from build123d import *

# Parameters (mm, degrees)
SKETCH1_R           = 2
BOSS_EXTRUDE1_DEPTH = 3
SKETCH2_R           = 5.5
SKETCH2_R_2         = 4
BOSS_EXTRUDE2_DEPTH = 0.5
SKETCH4_R           = 4
CUT_EXTRUDE2_DEPTH  = 7


with BuildPart() as part:
    # Sketch1 → Boss-Extrude1 (new body, symmetric)
    with BuildSketch(Plane.XY):
        with BuildLine():
            Line((-5.5, 0), (-14.456832295, -4))
            ThreePointArc((-14.456832295, -4), (0, -15), (14.456832295, -4))
            Line((14.456832295, -4), (5.5, 0))
            ThreePointArc((5.5, 0), (5.475559526, 0.517926522), (5.402455316, 1.03125))
            Line((5.402455316, 1.03125), (3.929058411, 8.75))
            ThreePointArc((3.929058411, 8.75), (0, 12), (-3.929058411, 8.75))
            Line((-3.929058411, 8.75), (-5.402455316, 1.03125))
            ThreePointArc((-5.402455316, 1.03125), (-5.475559526, 0.517926522), (-5.5, 0))
        make_face()
        with Locations((0, 8)):
            Circle(SKETCH1_R, mode=Mode.SUBTRACT)
    extrude(amount=BOSS_EXTRUDE1_DEPTH, both=True)

    # Sketch2 → Boss-Extrude2 (add)
    with BuildSketch(Plane.XY.offset(3)):
        Circle(SKETCH2_R)
        Circle(SKETCH2_R_2, mode=Mode.SUBTRACT)
    extrude(amount=BOSS_EXTRUDE2_DEPTH)

    # Sketch4 → Cut-Extrude2 (cut, through all)
    with BuildSketch(Plane.XY.offset(3)):
        Circle(SKETCH4_R)
    extrude(amount=-CUT_EXTRUDE2_DEPTH, mode=Mode.SUBTRACT)

    # Sketch8 → M4 Tapped Hole1 (revolve, cut)
    with BuildSketch(Plane(origin=(0, 0, 0), x_dir=(0, 0, 1), z_dir=(1, 0, 0))):
        Polygon((0, 0), (0, 22.491420021), (1.65, 21.5), (1.65, 0), align=None)
    revolve(axis=Axis((0, 6.35, 0), (0, -1, 0)), mode=Mode.SUBTRACT)


solid = part.part
Check sheet for the modelled part. Datum: model origin and axes. Units: mm. Give positions to 0.01 mm unless a question says otherwise; leave off trailing zeros. Loops run counter-clockwise (first coordinate to the right, second up) from the corner with the lowest first, then second, coordinate; pieces in that order, holes last. Notation, with made-up numbers: M 15,35 L 26,35 A12 ccw 26,51 Z; hole C 17.25,62 d5. An arc over 180 degrees is marked long. Return JSON: item names as keys, results as strings. Group by question number.
1. Cross-section at C-C on y = -0.75. Record the boundary of the cut face in (x, z), plus the area to 3 significant figures.
2. Cross-section at A-A on x = 0. Record the boundary of the cut face in (y, z), plus the area to 3 significant figures.
3. Mould release check, pull along Z, two halves, no side actions. Record for faces 1 (the flat face through (-0.2, -4.3, -3)), 2 (the cylindrical face through (-1.115, -9.244, -1.216)), 3 (the cylindrical face through (0, 10, 0)), 4 (the flat face through (1, 6, 3)): released by +Z, released by -Z, zero draft, split by the parting line, or undercut.
4. Go/stop test with flat-tipped pins: pin 1 (1.5 mm diameter, centred on x = -3.5, z = 2.5, fed in from +Y); pin 2 (1.5 mm diameter, centred on x = -4.5, z = 1.5, fed in from -Y); pin 3 (4.5 mm diameter, centred on x = -7, y = -10.5, fed in from +Z); pin 4 (6.5 mm diameter, centred on x = 0, y = 0, fed in from +Z). Record where each tip stops, or that it passes through.
5. Cross-section at D-D on z = 0. Record the boundary of the cut face in (x, y).
6. Cross-section at B-B on z = 2.25. Record the boundary of the cut face in (x, y).
7. Thickness scan on L1, parallel to Y at x = 0.5, z = -2.5; L2, parallel to Z at x = 0, y = -9.75; L3, parallel to Y at x = 0, z = -0.35. Record the ranges inside material, lowest first.
Return value:
{
 "1": {"outline": "M -7.18,-3 L -3.93,-3 L -3.93,3.5 L -5.45,3.5 L -5.45,3 L -7.18,3 Z; M 3.93,-3 L 7.18,-3 L 7.18,3 L 5.45,3 L 5.45,3.5 L 3.93,3.5 Z", "area": "40.5 mm^2"},
 "2": {"outline": "M -15,-3 L -4,-3 L -4,-1.65 L -15,-1.65 Z; M -15,1.65 L -4,1.65 L -4,3.5 L -5.5,3.5 L -5.5,3 L -15,3 Z; M 4,-3 L 6,-3 L 6,3 L 5.5,3 L 5.5,3.5 L 4,3.5 Z; M 10,-3 L 12,-3 L 12,3 L 10,3 Z", "area": "55.2 mm^2"},
 "3": {"face 1": "released by -Z", "face 2": "undercut", "face 3": "zero draft", "face 4": "released by +Z"},
 "4": {"pin 1": "y = 10.9", "pin 2": "y = -14.52", "pin 3": "z = 3", "pin 4": "through"},
 "5": {"outline": "M -14.46,-4 A15 ccw -1.65,-14.91 L -1.65,-3.64 A4 cw long 1.65,-3.64 L 1.65,-14.91 A15 ccw 14.46,-4 L 5.5,0 A5.5 ccw 5.4,1.03 L 3.93,8.75 A4 ccw -3.93,8.75 L -5.4,1.03 A5.5 ccw -5.5,0 Z; hole C 0,8 d4"},
 "6": {"outline": "M -14.46,-4 A15 ccw 14.46,-4 L 5.5,0 A5.5 ccw 5.4,1.03 L 3.93,8.75 A4 ccw -3.93,8.75 L -5.4,1.03 A5.5 ccw -5.5,0 Z; hole C 0,0 d8; hole C 0,8 d4"},
 "7": {"L1": "-14.99 to -3.97, 3.97 to 6.06, 9.94 to 11.97", "L2": "-3 to -1.65, 1.65 to 3", "L3": "4 to 6, 10 to 12"}
}
